```python
from build123d import *

# Parameters (mm, degrees)
BOSS_EXTRUDE1_DEPTH               = 95
SKETCH2_R                         = 2
CUT_EXTRUDE1_DEPTH                = 143.06424603
ESQUISSE2_R                       = 2
ENL_V_MAT_EXTRU_2_DEPTH           = 143.06424603
ESQUISSE3_R                       = 4
ENL_V_MAT_EXTRU_3CNC_DEPTH        = 143.06424603
ESQUISSE4_R                       = 1.5
ENL_V_MAT_EXTRU_4_3DPRINTER_DEPTH = 143.06424603


with BuildPart() as part:
    # Sketch1 → Boss-Extrude1 (new body)
    with BuildSketch(Plane.XY):
        with BuildLine():
            Line((0, -19.651530772), (0, 0))
            Line((0, 0), (-11.5, 0))
            Line((-11.5, 0), (-11.5, -52.5))
            Line((-11.5, -52.5), (0, -52.5))
            Line((0, -52.5), (0, -34.348469228))
            ThreePointArc((0, -34.348469228), (-6, -27), (0, -19.651530772))
        make_face()
        with BuildLine():
            Line((0, -52.5), (-11.5, -52.5))
            Line((-11.5, -52.5), (-11.5, -105))
            Line((-11.5, -105), (0, -105))
            Line((0, -105), (0, -85.348469228))
            ThreePointArc((0, -85.348469228), (-6, -78), (0, -70.651530772))
            Line((0, -70.651530772), (0, -52.5))
        make_face()
    extrude(amount=BOSS_EXTRUDE1_DEPTH)

    # Sketch2 → Cut-Extrude1 (cut, through all)
    with BuildSketch(Plane(origin=(0, 0, 0), x_dir=(0, 0, -1), z_dir=(1, 0, 0))):
        with Locations(Location((-83, -100, 0), (0, 0, 90))):
            Circle(SKETCH2_R)
        with Locations(Location((-12, -100, 0), (0, 0, 270))):
            Circle(SKETCH2_R)
    extrude(amount=-CUT_EXTRUDE1_DEPTH, mode=Mode.SUBTRACT)

    # Esquisse2 → Enlèv. mat.-Extru.2 (cut, through all)
    with BuildSketch(Plane(origin=(0, 0, 0), x_dir=(0, 0, -1), z_dir=(1, 0, 0))):
        with Locations(Location((-6, -39.5, 0), (0, 0, 90))):
            Circle(ESQUISSE2_R)
        with Locations(Location((-89, -39.5, 0), (0, 0, 90))):
            Circle(ESQUISSE2_R)
    extrude(amount=-ENL_V_MAT_EXTRU_2_DEPTH, mode=Mode.SUBTRACT)

    # Esquisse3 → Enlèv. mat.-Extru.3CNC (cut, through all)
    with BuildSketch(Plane.ZY.offset(11.5)):
        with Locations((80, -10)):
            Circle(ESQUISSE3_R)
        with Locations((15, -10)):
            Circle(ESQUISSE3_R)
        with Locations((72.5, -92)):
            Circle(ESQUISSE3_R)
        with Locations((22.5, -92)):
            Circle(ESQUISSE3_R)
    extrude(amount=-ENL_V_MAT_EXTRU_3CNC_DEPTH, mode=Mode.SUBTRACT)

    # Esquisse4 → Enlèv. mat.-Extru.4-3Dprinter (cut, through all)
    with BuildSketch(Plane(origin=(0, 0, 0), x_dir=(0, 0, -1), z_dir=(1, 0, 0))):
        with Locations(Location((-32.5, -10, 0), (0, 0, 90))):
            Circle(ESQUISSE4_R)
        with Locations(Location((-63.5, -10, 0), (0, 0, 90))):
            Circle(ESQUISSE4_R)
        with Locations(Location((-63.5, -41, 0), (0, 0, 90))):
            Circle(ESQUISSE4_R)
        with Locations(Location((-32.5, -41, 0), (0, 0, 90))):
            Circle(ESQUISSE4_R)
        with Locations(Location((-40.5, -65, 0), (0, 0, 90))):
            Circle(ESQUISSE4_R)
        with Locations(Location((-63.5, -65, 0), (0, 0, 90))):
            Circle(ESQUISSE4_R)
    extrude(amount=-ENL_V_MAT_EXTRU_4_3DPRINTER_DEPTH, mode=Mode.SUBTRACT)


solid = part.part
```
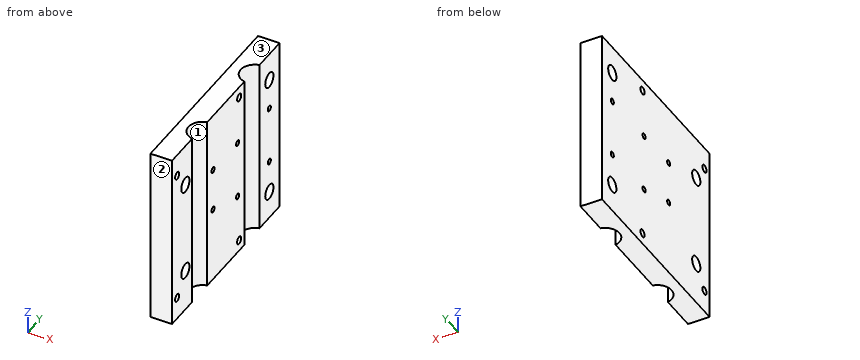
Geometry: final body of the model. Coordinates: model frame, mm. Face numbers are marked on the shaded views. Round coordinates to 2 decimals unless told otherwise and drop trailing zeros. Loops run counter-clockwise (first coordinate to the right, second up) from the corner with the lowest first, then second, coordinate; pieces in that order, holes last. Notation, with made-up numbers: (31, 26) -> (59, 26) arc R11 cw to (59, 31) -> close; hole circle Ø1 at (51.5, 30.5). An arc over 180 degrees is marked (long way). Use one line per item in the form item = value. Start each with the question number.
1) Draft query along Y for the marked faces 1, 2 and 3. Return one class per face: released by +Y, released by -Y, zero draft, split by the parting line, or undercut.
2) Line query: L1, parallel to Z at x = -10.25, y = -100; L2, parallel to Z at x = -9.5, y = -9; L3, parallel to Y at x = -8.25, z = 15. Output: solid intervals per line, ascending.
3) Section A-A on z = 40.5. Output: boundary loops of the cut face in (x, y), then the cut area to 3 significant figures.
4) Section D-D on z = 63.5. Output: boundary loops of the cut face in (x, y).
5) Section C-C on x = -2.75. Give the number of separate pieces and of enclosed holes in the cut face, then the cut area to 3 significant figures.
6) Section B-B on y = -92. Output: boundary loops of the cut face in (x, z).
Response:
q1.face_1 = undercut
q1.face_2 = released by -Y
q1.face_3 = zero draft
q2.L1 = 0 to 10, 14 to 81, 85 to 95
q2.L2 = 0 to 11.13, 18.87 to 31.38, 33.62 to 62.38, 64.62 to 76.13, 83.87 to 95
q2.L3 = -105 to -14, -6 to 0
q3.outline = (-11.5, -105) -> (0, -105) -> (0, -85.35) arc R7.5 cw to (0, -70.65) -> (0, -66.5) -> (-11.5, -66.5) -> close; (-11.5, -63.5) -> (0, -63.5) -> (0, -34.35) arc R7.5 cw to (0, -19.65) -> (0, 0) -> (-11.5, 0) -> close
q3.area = 1,040 mm^2
q4.outline = (-11.5, -105) -> (0, -105) -> (0, -85.35) arc R7.5 cw to (0, -70.65) -> (0, -66.5) -> (-11.5, -66.5) -> close; (-11.5, -63.5) -> (0, -63.5) -> (0, -42.5) -> (-11.5, -42.5) -> close; (-11.5, -39.5) -> (0, -39.5) -> (0, -34.35) arc R7.5 cw to (0, -19.65) -> (0, -11.5) -> (-11.5, -11.5) -> close; (-11.5, -8.5) -> (0, -8.5) -> (0, 0) -> (-11.5, 0) -> close
q5.separate_pieces = 3
q5.enclosed_holes = 14
q5.area = 7,330 mm^2
q6.outline = (-11.5, 0) -> (0, 0) -> (0, 18.5) -> (-11.5, 18.5) -> close; (-11.5, 26.5) -> (0, 26.5) -> (0, 68.5) -> (-11.5, 68.5) -> close; (-11.5, 76.5) -> (0, 76.5) -> (0, 95) -> (-11.5, 95) -> close
